Read the model definition and answer for the solid it produces. Units are mm, in the model's axes. A direction names the side the tool comes from. Coordinates: 2 decimals unless noted, no trailing zeros. Loops run counter-clockwise (first coordinate to the right, second up) from the corner with the lowest first, then second, coordinate; pieces in that order, holes last. Notation, with made-up numbers: M -17,45 L 21,45 A11 cw 21,55 Z; hole C 4,7.25 d5. An arc over 180 degrees is marked long. Put each result on its own line as item: value.
from build123d import *

# Parameters (mm, degrees)
SKETCH1_W           = 132.08
SKETCH1_H           = 57.15
BOSS_EXTRUDE1_DEPTH = 6.35
SKETCH2_W           = 132.08
SKETCH2_H           = 6.35
BOSS_EXTRUDE2_DEPTH = 31.242
SKETCH3_W           = 132.08
SKETCH3_H           = 6.35
BOSS_EXTRUDE3_DEPTH = 180.34
SKETCH4_W           = 7.62
SKETCH4_H           = 186.69
BOSS_EXTRUDE4_DEPTH = 6.35
SKETCH5_W           = 147.32
SKETCH5_H           = 90.17
BOSS_EXTRUDE5_DEPTH = 2.54


with BuildPart() as part:
    # Sketch1 → Boss-Extrude1 (new body)
    with BuildSketch(Plane.XY):
        with Locations((35.892678297, -11.105284376)):
            Rectangle(SKETCH1_W, SKETCH1_H)
    extrude(amount=BOSS_EXTRUDE1_DEPTH)

    # Sketch2 → Boss-Extrude2 (add)
    with BuildSketch(Plane(origin=(0, 0, 0), x_dir=(-1, 0, 0), z_dir=(0, 0, -1))):
        with Locations((-35.892678297, 5.912715624)):
            Rectangle(SKETCH2_W, SKETCH2_H)
    extrude(amount=BOSS_EXTRUDE2_DEPTH)

    # Sketch3 → Boss-Extrude3 (add)
    with BuildSketch(Plane.XY.offset(6.35)):
        with Locations((35.892678297, -36.505284376)):
            Rectangle(SKETCH3_W, SKETCH3_H)
    extrude(amount=BOSS_EXTRUDE3_DEPTH)

    # Sketch4 → Boss-Extrude4 (add)
    with BuildSketch(Plane.XZ.offset(39.680284376)):
        with Locations((-33.957321703, 93.345)):
            Rectangle(SKETCH4_W, SKETCH4_H)
        with Locations((105.742678297, 93.345)):
            Rectangle(SKETCH4_W, SKETCH4_H)
    extrude(amount=-BOSS_EXTRUDE4_DEPTH)

    # Sketch5 → Boss-Extrude5 (add)
    with BuildSketch(Plane(origin=(0, -33.330284376, 0), x_dir=(1, 0, 0), z_dir=(0, 1, 0))):
        with Locations((35.892678297, -141.605)):
            Rectangle(SKETCH5_W, SKETCH5_H)
    extrude(amount=BOSS_EXTRUDE5_DEPTH)


solid = part.part
1) Find section A-A, the plane x = 57.5. Write down the section's boundary in (y, z).
Answer list:
outline: M -39.68,0 L 2.74,0 L 2.74,-31.24 L 9.09,-31.24 L 9.09,0 L 17.47,0 L 17.47,6.35 L -33.33,6.35 L -33.33,96.52 L -30.79,96.52 L -30.79,186.69 L -39.68,186.69 Z
2) Straight lines are drawn through the part: line 1 (Z direction, x = 69, y = 14.5); line 2 (Y direction, x = 40.5, z = 16); line 3 (Y direction, x = -29, z = -22). For each, find the intervals that lie inside material, in ascending order. Write a range as [from, to].
Answer list:
line 1: z = [0, 6.35]
line 2: y = [-39.68, -33.33]
line 3: y = [2.74, 9.09]
3) Given pin 1 Ø5 at (x, y) = (10.5, -18) entering from +Z; pin 2 Ø12.5 at (x, y) = (65, -29) entering from -Z; pin 3 Ø1 at (y, z) = (-30, 4) entering from -X, each flat-ended and moving along its own axis, determine where each tip first touches the part or whether it passes through.
Answer list:
pin 1: stops at z = 6.35
pin 2: stops at z = 0
pin 3: stops at x = -30.15
4) Find section C-C, the plane y = -2. Write down the section's boundary in (x, z), plus the area to 3 significant figures.
Answer list:
outline: M -30.15,0 L 101.93,0 L 101.93,6.35 L -30.15,6.35 Z
area: 839 mm^2
5) Find section B-B, the plane z = 117. Write down the section's boundary in (x, y).
Answer list:
outline: M -37.77,-39.68 L 109.55,-39.68 L 109.55,-30.79 L -37.77,-30.79 Z
6) Which of the six approach directions +Z, -Z, +X, -X, +Y, -Y give full straight-line access (tool end or side, diameter ignored) to faces 1 (the flat face through (35, -35, 186.69)), 2 (the flat face through (35, -19, 0)), 3 (the flat face through (37, 6, -31.242)), 4 (the flat face through (35, -30.79, 141)), 5 (the flat face through (37, 9.088, -15))?
Answer list:
face 1: +Z, +X, -X, +Y, -Y
face 2: -Z, +X, -X, -Y
face 3: -Z, +X, -X, +Y, -Y
face 4: +Z, +X, -X, +Y
face 5: -Z, +X, -X, +Y
